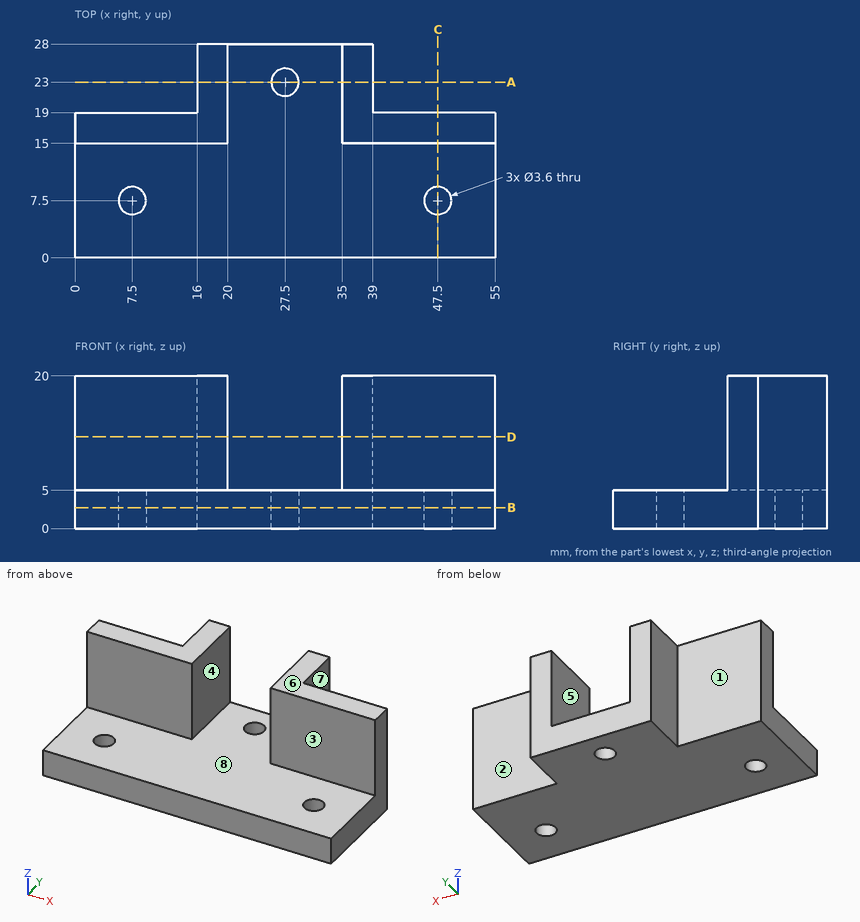
Study the drawing (mm; zero at the part's minimum x, y, z) and answer. A direction names the side the tool comes from. Round coordinates to 2 decimals unless told otherwise and drop trailing zeros. Order: outer loops, then holes, each group sorted by start corner. A loop starts at its lowest first (then second) coordinate and runs counter-clockwise, first axis right, second up. Notation, with made-up numbers: (-6, 73) - (28, 73) arc R29 cw to (28, 93) - close; hole circle Ø6 at (-25, 53.5). An arc over 180 degrees is marked (long way). Use one line per item in the form item = value. Start each with the question number.
(1) The part is cut by section C-C (x = 47.5). Give the vertices of the cut face in (y, z), then the cut area to 3 significant figures.
(2) The part is cut by section A-A (y = 23). Give the vertices of the cut face in (x, z), then the cut area to 3 significant figures.
(3) The part is cut by section D-D (z = 12). Give the vertices of the cut face in (x, y), then the cut area to 3 significant figures.
(4) Flat-ended cylindrical pins translate along their axes: pin 1 Ø5 at (y, z) = (15, 16) entering from -X; pin 2 Ø4.5 at (x, z) = (48, 10.5) entering from -Y; pin 3 Ø1 at (x, z) = (13.5, 17.5) entering from +Y; pin 4 Ø4.5 at (y, z) = (22, 7) entering from -X. Find the tip coordinate at first contact, or state that the pin passes through.
(5) Find the intervals of material crossed by line 1 along X through (y, z) = (22.75, 13.25); line 2 along Y through (x, z) = (7.5, 2.4); line 3 along Y through (x, z) = (5, 8.75), in increasing order. Write a range as from..to.
(6) The part is cut by section B-B (z = 2.75). Give the vertices of the cut face in (x, y), then the cut area to 3 significant figures.
(7) For the marked faces 1, 2, 3 and 4, determine the directions among +Z, -Z, +X, -X, +Y, -Y from which every point of the face is accessible in a straight line to the end or side of a thin tool.
(8) Determine the mould class of the marked faces 5, 6, 7 and 8 for opening direction X: +X half, -X half, draft (parallel to the pull), parting line (faces both ways), or undercut.
Checked values:
q1.outline = (0, 0) - (5.7, 0) - (5.7, 5) - (0, 5) - close; (9.3, 0) - (19, 0) - (19, 20) - (15, 20) - (15, 5) - (9.3, 5) - close
q1.area = 137 mm^2
q2.outline = (16, 0) - (25.7, 0) - (25.7, 5) - (20, 5) - (20, 20) - (16, 20) - close; (29.3, 0) - (39, 0) - (39, 20) - (35, 20) - (35, 5) - (29.3, 5) - close
q2.area = 217 mm^2
q3.outline = (0, 15) - (20, 15) - (20, 28) - (16, 28) - (16, 19) - (0, 19) - close; (35, 15) - (55, 15) - (55, 19) - (39, 19) - (39, 28) - (35, 28) - close
q3.area = 232 mm^2
q4.pin_1 = 0
q4.pin_2 = 15
q4.pin_3 = 19
q4.pin_4 = 16
q5.line_1 = 16..20, 35..39
q5.line_2 = 0..5.7, 9.3..19
q5.line_3 = 15..19
q6.outline = (0, 0) - (55, 0) - (55, 19) - (39, 19) - (39, 28) - (16, 28) - (16, 19) - (0, 19) - close; hole circle Ø3.6 at (7.5, 7.5); hole circle Ø3.6 at (27.5, 23); hole circle Ø3.6 at (47.5, 7.5)
q6.area = 1,220 mm^2
q7.face_1 = +Z, -Z, -X, +Y
q7.face_2 = +Z, -Z, +X, +Y
q7.face_3 = +Z, +X, -X, -Y
q7.face_4 = +Z, +Y, -Y
q8.face_5 = undercut
q8.face_6 = draft
q8.face_7 = +X half
q8.face_8 = undercut
